For this review, take the finished solid that the model builds, in its own axes (mm). Round coordinates to 2 decimals unless told otherwise and drop trailing zeros. Write each loop counter-clockwise with the first axis right and the second up, starting at its lowest first coordinate (ties: lowest second). Pieces come first, ordered by that corner, then holes. Notation, with made-up numbers: M -9.5,72.25 L 18.5,72.25 A22 cw 18.5,80.25 Z; hole C -18,62 d1. An arc over 180 degrees is marked long. Answer in a Markdown table with one row per item.
```python
from build123d import *

# Parameters (mm, degrees)
SKETCH1_R           = 1
SKETCH1_R_2         = 1.25
BOSS_EXTRUDE1_DEPTH = 2


with BuildPart() as part:
    # Sketch1 → Boss-Extrude1 (new body)
    with BuildSketch(Plane(origin=(0, 0, 0), x_dir=(0, 0, -1), z_dir=(1, 0, 0))):
        with BuildLine():
            ThreePointArc((-1.060660172, 3.889087297), (-3.889087297, 3.889087297), (-3.889087297, 1.060660172))
            Line((-3.889087297, 1.060660172), (1.414213562, -4.242640687))
            ThreePointArc((1.414213562, -4.242640687), (4.242640687, -4.242640687), (4.242640687, -1.414213562))
            Line((4.242640687, -1.414213562), (-1.060660172, 3.889087297))
        make_face()
        with Locations((2.828427125, -2.828427125)):
            Circle(SKETCH1_R, mode=Mode.SUBTRACT)
        Circle(SKETCH1_R_2, mode=Mode.SUBTRACT)
        with Locations((-2.474873734, 2.474873734)):
            Circle(SKETCH1_R, mode=Mode.SUBTRACT)
    extrude(amount=BOSS_EXTRUDE1_DEPTH)


solid = part.part
```
Q1. Take a section at B-B (y = 0). State the section outline as (x, z) points.
Found:
| item | result |
|---|---|
| outline | M 0,-2.83 L 2,-2.83 L 2,-1.25 L 0,-1.25 Z; M 0,1.25 L 2,1.25 L 2,2.83 L 0,2.83 Z |
Q2. Take a section at A-A (x = 1.55). State the section outline as (y, z) points, then the cut area to 3 significant figures.
Found:
| item | result |
|---|---|
| outline | M -4.24,-1.41 A2 ccw -1.41,-4.24 L 3.89,1.06 A2 ccw 1.06,3.89 Z; hole C -2.83,-2.83 d2; hole C 0,0 d2.5; hole C 2.47,2.47 d2 |
| area | 31.4 mm² |
Q3. Mouldability with a two-part tool opening along Y and no side actions: class faces 1 (the face through (0.99, 1.2, -1.63)), 2 (the face through (0.986, -4.273, -4.211)), 3 (the face through (1, -3.8, -2.6)), 4 (the face through (0.99, -1.22, 0.27)) as +Y half, -Y half, draft (parallel to the pull), parting line (faces both ways), or undercut.
Found:
| item | result |
|---|---|
| face 1 | +Y half |
| face 2 | parting line |
| face 3 | undercut |
| face 4 | undercut |
Q4. Insertion check: P1, Ø5, axis at y = -1.5, z = -2.5, coming from the -X side; P2, Ø1, axis at x = 1.5, y = 3, coming from the -Z side; P3, Ø1, axis at x = 1, z = -2, coming from the +Y side. Each pin has a flat end and moves straight along its axis. Give the tip position at first contact, or say it passes through.
Found:
| item | result |
|---|---|
| P1 | x = 0 |
| P2 | z = -0.33 |
| P3 | y = 1.33 |
Q5. For probe 1 along Y at (x, z) = (1, 2); probe 2 along Z at (x, y) = (1.9, 1.75); probe 3 along Z at (x, y) = (0.35, -2), list the stretches that pass through material, from the lowest coordinate up.
Found:
| item | result |
|---|---|
| probe 1 | -0.83 to 1.59, 3.35 to 4.42 |
| probe 2 | -1.08 to 1.79, 3.16 to 4.34 |
| probe 3 | -4.65 to -3.39, -2.27 to 0.83 |
